from build123d import *

# Parameters (mm, degrees)
SKETCH1_R               = 19.939
CIRCLE_EXTRUDE_DEPTH    = 7.62
SKETCH3_W               = 7.62
SKETCH3_H               = 39.878
RECTANGLE_EXTRUDE_DEPTH = 63.5
SKETCH2_R               = 18.034
CRICLE_CUT_DEPTH        = 67.991627245
SKETCH4_OUTSIDE_W       = 103.997
SKETCH4_OUTSIDE_H       = 60.436
SKETCH4_OUTSIDE_W_2     = 61.595
SKETCH4_OUTSIDE_H_2     = 36.068
FRAME_CUT_DEPTH         = 67.991627245
EXTENSION_DEPTH         = 2.54
SKETCH11_W              = 5.08
SKETCH11_H              = 36.068
MIDDLE_DEPTH            = 46.682766784
SKETCH12_OUTSIDE_W      = 78.015
SKETCH12_OUTSIDE_H      = 52.488
CIRCLE_EXTENSION_DEPTH  = 5.08


with BuildPart() as part:
    # Sketch1 → circle extrude (new body)
    with BuildSketch(Plane.XY):
        with Locations(Location((0, 0, 0), (0, 0, 180))):
            Circle(SKETCH1_R)
    extrude(amount=CIRCLE_EXTRUDE_DEPTH)

    # Sketch3 → rectangle extrude (add)
    with BuildSketch(Plane(origin=(0, 0, 0), x_dir=(0, 0, -1), z_dir=(1, 0, 0))):
        with Locations((-3.81, 0)):
            Rectangle(SKETCH3_W, SKETCH3_H)
    extrude(amount=RECTANGLE_EXTRUDE_DEPTH)

    # Sketch2 → cricle cut (cut, through all)
    with BuildSketch(Plane.XY.offset(7.62)):
        Circle(SKETCH2_R)
    extrude(amount=-CRICLE_CUT_DEPTH, mode=Mode.SUBTRACT)

    # Sketch4 outside → frame cut (cut, through all)
    with BuildSketch(Plane.XY.offset(7.62)):
        with Locations((21.7805, 0)):
            Rectangle(SKETCH4_OUTSIDE_W, SKETCH4_OUTSIDE_H)
        with Locations((30.7975, 0)):
            Rectangle(SKETCH4_OUTSIDE_W_2, SKETCH4_OUTSIDE_H_2, mode=Mode.SUBTRACT)
    extrude(amount=-FRAME_CUT_DEPTH, mode=Mode.SUBTRACT)

    # Sketch10 → extension (add)
    with BuildSketch(Plane(origin=(0, 0, 0), x_dir=(-1, 0, 0), z_dir=(0, 0, -1))):
        with BuildLine():
            Line((0, 18.034), (-61.595, 18.034))
            Line((-61.595, 18.034), (-61.595, -18.034))
            Line((-61.595, -18.034), (0, -18.034))
            ThreePointArc((0, -18.034), (-18.034, 0), (0, 18.034))
        make_face()
    extrude(amount=EXTENSION_DEPTH)

    # Sketch11 → middle (cut, through all)
    with BuildSketch(Plane(origin=(20.32, 0, 0), x_dir=(0, 0, -1), z_dir=(1, 0, 0))):
        with Locations((-2.54, 0)):
            Rectangle(SKETCH11_W, SKETCH11_H)
    extrude(amount=MIDDLE_DEPTH, mode=Mode.SUBTRACT)

    # Sketch12 outside → circle extension (cut)
    with BuildSketch(Plane.XY):
        with Locations((30.7975, 0)):
            Rectangle(SKETCH12_OUTSIDE_W, SKETCH12_OUTSIDE_H)
        with BuildLine():
            Line((2.286, 18.034), (0, 18.034))
            Line((0, 18.034), (0, -18.034))
            Line((0, -18.034), (2.286, -18.034))
            ThreePointArc((2.286, -18.034), (20.32, 0), (2.286, 18.034))
        make_face(mode=Mode.SUBTRACT)
    extrude(amount=CIRCLE_EXTENSION_DEPTH, mode=Mode.SUBTRACT)


solid = part.part
Read the model definition and answer for the solid it produces. Units are mm, in the model's axes. A direction names the side the tool comes from. Give positions to 0.01 mm unless a question says otherwise; leave off trailing zeros. Write each loop counter-clockwise with the first axis right and the second up, starting at its lowest first coordinate (ties: lowest second). Pieces come first, ordered by that corner, then holes. Notation, with made-up numbers: (57.5, -27.5) - (82.5, -27.5) arc R9 cw to (82.5, -22.5) - close; hole circle Ø9 at (-5, 8). An arc over 180 degrees is marked (long way). Return JSON: item names as keys, results as strings.
Q1. For faces 1 (the face through (37, 0, 7.62)), 2 (the face through (20.316, -0.397, 2.504)), determine the directions among +Z, -Z, +X, -X, +Y, -Y from which every point of the face is accessible in a straight line to the end or side of a thin tool.
Reply:
{"face 1": "+Z, +X, -X, +Y, -Y", "face 2": "+X"}
Q2. For a pull along Z with two mould halves and no side action, classify faces 3 (the face through (30, 18.034, 6)), 4 (the face through (38, 0, -2.54)), 5 (the face through (38, 0, 5.08)) as released by +Z, released by -Z, zero draft, split by the parting line, or undercut.
Reply:
{"face 3": "zero draft", "face 4": "released by -Z", "face 5": "undercut"}
Q3. Given P1, Ø6, axis at x = 48, z = 4.5, coming from the -Y side; P2, Ø2, axis at y = -7, z = 4.5, coming from the -X side, each flat-ended and moving along its own axis, determine where each tip first touches the part or whether it passes through.
Reply:
{"P1": "y = -18.03", "P2": "x = 16.16"}
Q4. A cutting plane is placed at A-A, the plane x = 27. Determine the outline of the cut face in (y, z).
Reply:
{"outline": "(-18.03, -2.54) - (18.03, -2.54) - (18.03, 0) - (-18.03, 0) - close; (-18.03, 5.08) - (18.03, 5.08) - (18.03, 7.62) - (-18.03, 7.62) - close"}
Q5. A cutting plane is placed at D-D, the plane x = 13.5. Determine the outline of the cut face in (y, z), and give its area (3 significant figures).
Reply:
{"outline": "(-18.03, -2.54) - (-11.96, -2.54) - (-11.96, 7.62) - (-18.03, 7.62) - (-18.03, 5.08) - (-14.12, 5.08) - (-14.12, 0) - (-18.03, 0) - close; (11.96, -2.54) - (18.03, -2.54) - (18.03, 0) - (14.12, 0) - (14.12, 5.08) - (18.03, 5.08) - (18.03, 7.62) - (11.96, 7.62) - close", "area": "83.7 mm²"}
Q6. A cutting plane is placed at B-B, the plane y = -1. Determine the outline of the cut face in (x, z) (3 decimals), and give its area (3 significant figures).
Reply:
{"outline": "(18.006, -2.54) - (61.595, -2.54) - (61.595, 0) - (20.292, 0) - (20.292, 5.08) - (61.595, 5.08) - (61.595, 7.62) - (18.006, 7.62) - close", "area": "233 mm²"}
Q7. A cutting plane is placed at C-C, the plane z = 6.5. Determine the outline of the cut face in (x, y) (3 decimals).
Reply:
{"outline": "(0, -18.034) - (61.595, -18.034) - (61.595, 18.034) - (0, 18.034) arc R18.034 cw to start"}
Q8. Consider line 1 along Z through (x, y) = (34.5, 2); line 2 along Y through (x, z) = (16.5, 7); line 3 along Y through (x, z) = (11.5, 2.5). Determine where each line is inside the solid, lowest interval first. Write a range as [from, to].
Reply:
{"line 1": "[-2.54, 0], [5.08, 7.62]", "line 2": "[-18.03, -7.28], [7.28, 18.03]", "line 3": "[-15.5, -13.89], [13.89, 15.5]"}
